Verification items for the finished model (mm, model axes). Face numbers are marked on the shaded views. Round coordinates to 2 decimals unless told otherwise and drop trailing zeros. Write each loop counter-clockwise with the first axis right and the second up, starting at its lowest first coordinate (ties: lowest second). Pieces come first, ordered by that corner, then holes. Notation, with made-up numbers: (50, 52) -> (87, 52) arc R12 cw to (87, 59) -> close; hole circle Ø3 at (19.25, 14). An arc over 180 degrees is marked (long way). Use CSV: the item, a comma, the result in double quotes.
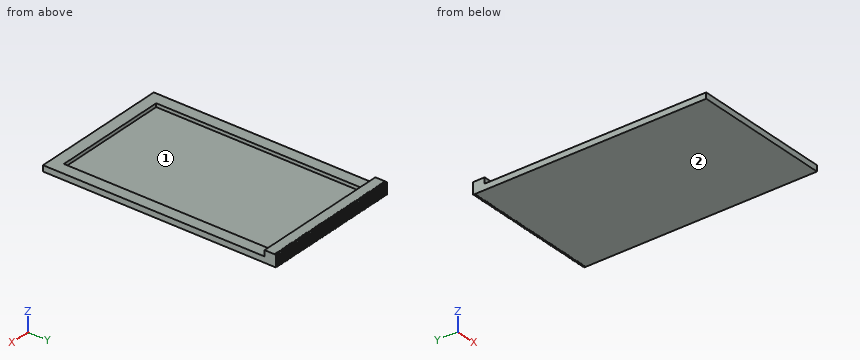
```python
from build123d import *

# Parameters (mm, degrees)
CROQUIS2_W              = 120
CROQUIS2_H              = 200
SALIENTE_EXTRUIR1_DEPTH = 5
CROQUIS3_W              = 100
CROQUIS3_H              = 180
CORTAR_EXTRUIR1_DEPTH   = 3
CROQUIS4_W              = 120
CROQUIS4_H              = 10
SALIENTE_EXTRUIR3_DEPTH = 5
CORTAR_EXTRUIR2_DEPTH   = 10
CROQUIS6_W              = 5
CROQUIS6_H              = 10
SALIENTE_EXTRUIR4_DEPTH = 120
CORTAR_EXTRUIR3_DEPTH   = 10


with BuildPart() as part:
    # Croquis2 → Saliente-Extruir1 (new body)
    with BuildSketch(Plane.XY):
        Rectangle(CROQUIS2_W, CROQUIS2_H)
    extrude(amount=SALIENTE_EXTRUIR1_DEPTH)

    # Croquis3 → Cortar-Extruir1 (cut)
    with BuildSketch(Plane.XY.offset(5)):
        Rectangle(CROQUIS3_W, CROQUIS3_H)
    extrude(amount=-CORTAR_EXTRUIR1_DEPTH, mode=Mode.SUBTRACT)

    # Croquis4 → Saliente-Extruir3 (add)
    with BuildSketch(Plane.XY.offset(5)):
        with Locations((0, 95)):
            Rectangle(CROQUIS4_W, CROQUIS4_H)
    extrude(amount=SALIENTE_EXTRUIR3_DEPTH)

    # Croquis5 → Cortar-Extruir2 (cut)
    with BuildSketch(Plane(origin=(0, 100, 0), x_dir=(1, 0, 0), z_dir=(0, 1, 0))):
        Polygon((59, -8), (58, -10), (60, -10), align=None)
        Polygon((57, -8), (56, -10), (58, -10), align=None)
        Polygon((55, -8), (54, -10), (56, -10), align=None)
        Polygon((53, -8), (52, -10), (54, -10), align=None)
        Polygon((51, -8), (50, -10), (52, -10), align=None)
        Polygon((49, -8), (48, -10), (50, -10), align=None)
        Polygon((47, -8), (46, -10), (48, -10), align=None)
        Polygon((45, -8), (44, -10), (46, -10), align=None)
        Polygon((43, -8), (42, -10), (44, -10), align=None)
        Polygon((41, -8), (40, -10), (42, -10), align=None)
        Polygon((39, -8), (38, -10), (40, -10), align=None)
        Polygon((37, -8), (36, -10), (38, -10), align=None)
        Polygon((35, -8), (34, -10), (36, -10), align=None)
        Polygon((33, -8), (32, -10), (34, -10), align=None)
        Polygon((31, -8), (30, -10), (32, -10), align=None)
        Polygon((29, -8), (28, -10), (30, -10), align=None)
        Polygon((27, -8), (26, -10), (28, -10), align=None)
        Polygon((25, -8), (24, -10), (26, -10), align=None)
        Polygon((23, -8), (22, -10), (24, -10), align=None)
        Polygon((21, -8), (20, -10), (22, -10), align=None)
        Polygon((19, -8), (18, -10), (20, -10), align=None)
        Polygon((17, -8), (16, -10), (18, -10), align=None)
        Polygon((15, -8), (14, -10), (16, -10), align=None)
        Polygon((13, -8), (12, -10), (14, -10), align=None)
        Polygon((11, -8), (10, -10), (12, -10), align=None)
        Polygon((9, -8), (8, -10), (10, -10), align=None)
        Polygon((7, -8), (6, -10), (8, -10), align=None)
        Polygon((5, -8), (4, -10), (6, -10), align=None)
        Polygon((3, -8), (2, -10), (4, -10), align=None)
        Polygon((1, -8), (0, -10), (2, -10), align=None)
        Polygon((-1, -8), (-2, -10), (0, -10), align=None)
        Polygon((-3, -8), (-4, -10), (-2, -10), align=None)
        Polygon((-5, -8), (-6, -10), (-4, -10), align=None)
        Polygon((-7, -8), (-8, -10), (-6, -10), align=None)
        Polygon((-9, -8), (-10, -10), (-8, -10), align=None)
        Polygon((-11, -8), (-12, -10), (-10, -10), align=None)
        Polygon((-13, -8), (-14, -10), (-12, -10), align=None)
        Polygon((-15, -8), (-16, -10), (-14, -10), align=None)
        Polygon((-17, -8), (-18, -10), (-16, -10), align=None)
        Polygon((-19, -8), (-20, -10), (-18, -10), align=None)
        Polygon((-21, -8), (-22, -10), (-20, -10), align=None)
        Polygon((-23, -8), (-24, -10), (-22, -10), align=None)
        Polygon((-25, -8), (-26, -10), (-24, -10), align=None)
        Polygon((-27, -8), (-28, -10), (-26, -10), align=None)
        Polygon((-29, -8), (-30, -10), (-28, -10), align=None)
        Polygon((-31, -8), (-32, -10), (-30, -10), align=None)
        Polygon((-33, -8), (-34, -10), (-32, -10), align=None)
        Polygon((-35, -8), (-36, -10), (-34, -10), align=None)
        Polygon((-37, -8), (-38, -10), (-36, -10), align=None)
        Polygon((-39, -8), (-40, -10), (-38, -10), align=None)
        Polygon((-41, -8), (-42, -10), (-40, -10), align=None)
        Polygon((-43, -8), (-44, -10), (-42, -10), align=None)
        Polygon((-45, -8), (-46, -10), (-44, -10), align=None)
        Polygon((-47, -8), (-48, -10), (-46, -10), align=None)
        Polygon((-49, -8), (-50, -10), (-48, -10), align=None)
        Polygon((-51, -8), (-52, -10), (-50, -10), align=None)
        Polygon((-53, -8), (-54, -10), (-52, -10), align=None)
        Polygon((-55, -8), (-56, -10), (-54, -10), align=None)
        Polygon((-57, -8), (-58, -10), (-56, -10), align=None)
        Polygon((-59, -8), (-60, -10), (-58, -10), align=None)
    extrude(amount=-CORTAR_EXTRUIR2_DEPTH, mode=Mode.SUBTRACT)

    # Croquis6 → Saliente-Extruir4 (add)
    with BuildSketch(Plane.ZY.offset(60)):
        with Locations((7.5, 95)):
            Rectangle(CROQUIS6_W, CROQUIS6_H)
    extrude(amount=-SALIENTE_EXTRUIR4_DEPTH)

    # Croquis7 → Cortar-Extruir3 (cut)
    with BuildSketch(Plane.XY.offset(10)):
        Polygon((-58, 100), (-60, 100), (-59, 98), align=None)
        Polygon((60, 100), (58, 100), (59, 98), align=None)
        Polygon((58, 100), (56, 100), (57, 98), align=None)
        Polygon((56, 100), (54, 100), (55, 98), align=None)
        Polygon((54, 100), (52, 100), (53, 98), align=None)
        Polygon((52, 100), (50, 100), (51, 98), align=None)
        Polygon((50, 100), (48, 100), (49, 98), align=None)
        Polygon((48, 100), (46, 100), (47, 98), align=None)
        Polygon((46, 100), (44, 100), (45, 98), align=None)
        Polygon((44, 100), (42, 100), (43, 98), align=None)
        Polygon((42, 100), (40, 100), (41, 98), align=None)
        Polygon((40, 100), (38, 100), (39, 98), align=None)
        Polygon((38, 100), (36, 100), (37, 98), align=None)
        Polygon((36, 100), (34, 100), (35, 98), align=None)
        Polygon((34, 100), (32, 100), (33, 98), align=None)
        Polygon((32, 100), (30, 100), (31, 98), align=None)
        Polygon((30, 100), (28, 100), (29, 98), align=None)
        Polygon((28, 100), (26, 100), (27, 98), align=None)
        Polygon((26, 100), (24, 100), (25, 98), align=None)
        Polygon((24, 100), (22, 100), (23, 98), align=None)
        Polygon((22, 100), (20, 100), (21, 98), align=None)
        Polygon((20, 100), (18, 100), (19, 98), align=None)
        Polygon((18, 100), (16, 100), (17, 98), align=None)
        Polygon((16, 100), (14, 100), (15, 98), align=None)
        Polygon((14, 100), (12, 100), (13, 98), align=None)
        Polygon((12, 100), (10, 100), (11, 98), align=None)
        Polygon((10, 100), (8, 100), (9, 98), align=None)
        Polygon((8, 100), (6, 100), (7, 98), align=None)
        Polygon((6, 100), (4, 100), (5, 98), align=None)
        Polygon((4, 100), (2, 100), (3, 98), align=None)
        Polygon((2, 100), (0, 100), (1, 98), align=None)
        Polygon((0, 100), (-2, 100), (-1, 98), align=None)
        Polygon((-2, 100), (-4, 100), (-3, 98), align=None)
        Polygon((-4, 100), (-6, 100), (-5, 98), align=None)
        Polygon((-6, 100), (-8, 100), (-7, 98), align=None)
        Polygon((-8, 100), (-10, 100), (-9, 98), align=None)
        Polygon((-10, 100), (-12, 100), (-11, 98), align=None)
        Polygon((-12, 100), (-14, 100), (-13, 98), align=None)
        Polygon((-14, 100), (-16, 100), (-15, 98), align=None)
        Polygon((-16, 100), (-18, 100), (-17, 98), align=None)
        Polygon((-18, 100), (-20, 100), (-19, 98), align=None)
        Polygon((-20, 100), (-22, 100), (-21, 98), align=None)
        Polygon((-22, 100), (-24, 100), (-23, 98), align=None)
        Polygon((-24, 100), (-26, 100), (-25, 98), align=None)
        Polygon((-26, 100), (-28, 100), (-27, 98), align=None)
        Polygon((-28, 100), (-30, 100), (-29, 98), align=None)
        Polygon((-30, 100), (-32, 100), (-31, 98), align=None)
        Polygon((-32, 100), (-34, 100), (-33, 98), align=None)
        Polygon((-34, 100), (-36, 100), (-35, 98), align=None)
        Polygon((-36, 100), (-38, 100), (-37, 98), align=None)
        Polygon((-38, 100), (-40, 100), (-39, 98), align=None)
        Polygon((-40, 100), (-42, 100), (-41, 98), align=None)
        Polygon((-42, 100), (-44, 100), (-43, 98), align=None)
        Polygon((-44, 100), (-46, 100), (-45, 98), align=None)
        Polygon((-46, 100), (-48, 100), (-47, 98), align=None)
        Polygon((-48, 100), (-50, 100), (-49, 98), align=None)
        Polygon((-50, 100), (-52, 100), (-51, 98), align=None)
        Polygon((-52, 100), (-54, 100), (-53, 98), align=None)
        Polygon((-54, 100), (-56, 100), (-55, 98), align=None)
        Polygon((-56, 100), (-58, 100), (-57, 98), align=None)
    extrude(amount=-CORTAR_EXTRUIR3_DEPTH, mode=Mode.SUBTRACT)


solid = part.part
```
Q1. Go/stop test with a flat-tipped pin: P1, Ø3, axis at x = -14, y = 33, coming from the +Z side. Record where the tip stops, or that it passes through.
Filled in:
P1,"z = 2"
Q2. Section check A-A (y = 60). Record the cut outline in (x, z), plus the area to 3 significant figures.
Filled in:
outline,"(-60, 0) -> (60, 0) -> (60, 5) -> (50, 5) -> (50, 2) -> (-50, 2) -> (-50, 5) -> (-60, 5) -> close"
area,"300 mm²"
Q3. Mould release check, pull along Y, two halves, no side actions. Record for the marked faces 1 and 2: released by +Y, released by -Y, zero draft, split by the parting line, or undercut.
Filled in:
face 1,"undercut"
face 2,"zero draft"
Q4. Material ranges on L1, parallel to Y at x = -4, z = 4.5; L2, parallel to X at y = 5, z = 2.25; L3, parallel to Y at x = 31, z = 3.5, recorded low to high.
Filled in:
L1,"-100 to -90, 90 to 100"
L2,"-60 to -50, 50 to 60"
L3,"-100 to -90, 90 to 98"
